Verification items for the finished model (mm, model axes). A direction names the side the tool comes from. Round coordinates to 2 decimals unless told otherwise and drop trailing zeros. Write each loop counter-clockwise with the first axis right and the second up, starting at its lowest first coordinate (ties: lowest second). Pieces come first, ordered by that corner, then holes. Notation, with made-up numbers: M 7.25,-19.5 L 60.25,-19.5 A13 cw 60.25,-1.5 Z; hole C 51.5,-13.75 d2. An arc over 180 degrees is marked long. One line per item, written item: value. Start each with the question number.
from build123d import *

# Parameters (mm, degrees)
BOSS_EXTRUDE1_DEPTH = 8
FILLET3_SIZE        = 7
SKETCH2_W           = 10
SKETCH2_H           = 8
CUT_EXTRUDE1_DEPTH  = 4
SKETCH3_R           = 3.5
CUT_EXTRUDE2_DEPTH  = 3


with BuildPart() as part:
    # Sketch1 → Boss-Extrude1 (new body)
    with BuildSketch(Plane.XY):
        Polygon((-6, -12), (-6, 12), (27, 12), (27, 17), (30, 17), (30, -17), (27, -17), (27, -12), align=None)
    extrude(amount=BOSS_EXTRUDE1_DEPTH)

    # Fillet3
    # a fillet whose section is not a circle: 7 mm, written as the material it takes off along each edge
    with BuildSketch(Plane(origin=(-6, 12, -17.5), x_dir=(0, -1, 0), z_dir=(0, 0, 1))) as fillet3_piece_1:
        with BuildLine():
            add(Edge.make_bspline([(FILLET3_SIZE, 0), (FILLET3_SIZE * 0.831801948466, 0), (FILLET3_SIZE * 0.663603896932, 0), (FILLET3_SIZE * 0.292893218813, FILLET3_SIZE * 0.0716919198361), (FILLET3_SIZE * 0.0716919198361, FILLET3_SIZE * 0.292893218813), (0, FILLET3_SIZE * 0.663603896932), (0, FILLET3_SIZE * 0.831801948466), (0, FILLET3_SIZE)], knots=[0, 0, 0, 0, 0, 0, 0.5, 0.5, 1, 1, 1, 1, 1, 1], degree=5))
            Line((0, FILLET3_SIZE), (0, 0))
            Line((0, 0), (FILLET3_SIZE, 0))
        make_face()
    extrude(amount=43, mode=Mode.SUBTRACT)
    with BuildSketch(Plane(origin=(-6, -12, -17.5), x_dir=(0, 1, 0), z_dir=(0, 0, 1))) as fillet3_piece_2:
        with BuildLine():
            add(Edge.make_bspline([(FILLET3_SIZE, 0), (FILLET3_SIZE * 0.831801948466, 0), (FILLET3_SIZE * 0.663603896932, 0), (FILLET3_SIZE * 0.292893218813, -FILLET3_SIZE * 0.0716919198361), (FILLET3_SIZE * 0.0716919198361, -FILLET3_SIZE * 0.292893218813), (0, -FILLET3_SIZE * 0.663603896932), (0, -FILLET3_SIZE * 0.831801948466), (0, -FILLET3_SIZE)], knots=[0, 0, 0, 0, 0, 0, 0.5, 0.5, 1, 1, 1, 1, 1, 1], degree=5))
            Line((0, -FILLET3_SIZE), (0, 0))
            Line((0, 0), (FILLET3_SIZE, 0))
        make_face()
    extrude(amount=43, mode=Mode.SUBTRACT)

    # Sketch2 → Cut-Extrude1 (cut)
    with BuildSketch(Plane.XY.offset(8)):
        with Locations((22, 4)):
            Rectangle(SKETCH2_W, SKETCH2_H)
        with Locations((22, -4)):
            Rectangle(SKETCH2_W, SKETCH2_H)
    extrude(amount=-CUT_EXTRUDE1_DEPTH, mode=Mode.SUBTRACT)

    # Sketch3 → Cut-Extrude2 (cut)
    with BuildSketch(Plane(origin=(30, 0, 0), x_dir=(0, 0, -1), z_dir=(1, 0, 0))):
        with Locations(Location((-4, 0, 0), (0, 0, 90))):
            Circle(SKETCH3_R)
    extrude(amount=-CUT_EXTRUDE2_DEPTH, mode=Mode.SUBTRACT)


solid = part.part
1) Access from +Z, -Z, +X, -X, +Y, -Y to the whole of each face (thin tool, end or side, straight path). Record for faces 4 (the cylindrical face through (28.521, -0.759, 0.583)), 5 (the flat face through (27, -0.1, 7.8)), 6 (the flat face through (14, 12, 4)).
2) Cross-section at C-C (y = 13.5). Record the boundary of the cut face in (x, z), then the cut area to 3 significant figures.
3) Cross-section at D-D (x = 11). Record the boundary of the cut face in (y, z), then the cut area to 3 significant figures.
4) Cross-section at A-A (y = 0). Record the boundary of the cut face in (x, z).
5) Gauge pin test, flat ends, axial feed: pin 1 Ø2 at (x, z) = (24.5, 7) entering from -Y; pin 2 Ø3 at (x, y) = (23.5, 4) entering from +Z; pin 3 Ø2 at (x, z) = (5.5, 5.5) entering from +Y; pin 4 Ø4 at (y, z) = (-0.5, 2) entering from +X. Record the tip position at first contact, or that the pin passes through.
6) Thickness scan on line 1 (Y direction, x = 19, z = 5.75); line 2 (Y direction, x = 28.15, z = 4); line 3 (Z direction, x = 28.35, y = 0). Record the ranges inside material, lowest first.
7) Cross-section at B-B (x = 17.5). Record the boundary of the cut face in (y, z).
8) Mould release check, pull along Z, two halves, no side actions. Record for faces 1 (the flat face through (12, 0, 0)), 2 (the flat face through (29, -17, 4)), 3 (the flat face through (27, 0, 3)): pulls with the +Z half, pulls with the -Z half, needs draft (parallel to the pull), parting line crosses it, or undercut.
Results below:
1. face 4: +X
1. face 5: +Z
1. face 6: +Z, -Z, -X, +Y
2. outline: M 27,0 L 30,0 L 30,8 L 27,8 Z
2. area: 24.0 mm²
3. outline: M -12,0 L 12,0 L 12,8 L -12,8 Z
3. area: 192 mm²
4. outline: M -6,0 L 30,0 L 30,0.5 L 27,0.5 L 27,4 L 17,4 L 17,8 L -6,8 Z; M 27,7.5 L 30,7.5 L 30,8 L 27,8 Z
5. pin 1: stops at y = -12
5. pin 2: stops at z = 4
5. pin 3: stops at y = 12
5. pin 4: stops at x = 30
6. line 1: y = -12 to -8, 8 to 12
6. line 2: y = -17 to -3.5, 3.5 to 17
6. line 3: z = 0 to 0.5, 7.5 to 8
7. outline: M -12,0 L 12,0 L 12,8 L 8,8 L 8,4 L -8,4 L -8,8 L -12,8 Z
8. face 1: pulls with the -Z half
8. face 2: needs draft
8. face 3: undercut
